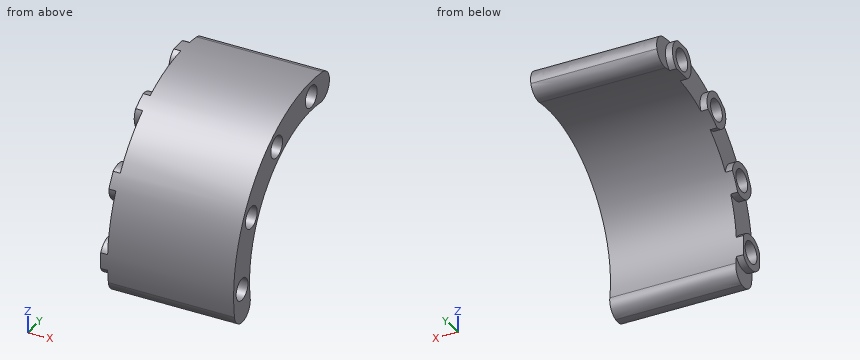
from build123d import *

# Parameters (mm, degrees)
SKETCH_1_R               = 41.5
SKETCH_1_R_2             = 33
EXTRUDE_1_DEPTH          = 38
SKETCH_2_R               = 3.15
CUT_EXTRUDE_1_DEPTH      = 70.91780889
PATTERN_CIRCULAR_1_COUNT = 4
PATTERN_CIRCULAR_1_ANGLE = 90
CUT_EXTRUDE_2_DEPTH      = 38
FILLET_START             = -1
FILLET_1_DEPTH           = 40
FILLET_2_DEPTH           = 38
SKETCH_4_OUTSIDE_W       = 69.583
SKETCH_4_OUTSIDE_H       = 69.583
SKETCH_4_OUTSIDE_R       = 5
CUT_EXTRUDE_3_DEPTH      = 2


with BuildPart() as part:
    # 草图1 → 凸台-拉伸1 (new body)
    with BuildSketch(Plane(origin=(0, 0, 0), x_dir=(0, 0, -1), z_dir=(1, 0, 0))):
        Circle(SKETCH_1_R)
        Circle(SKETCH_1_R_2, mode=Mode.SUBTRACT)
    extrude(amount=EXTRUDE_1_DEPTH)

    # 草图2 → 切除-拉伸1 (cut, through all)
    with BuildSketch(Plane.ZY):
        with Locations((37, 0)):
            Circle(SKETCH_2_R)
    cut_extrude_1 = extrude(amount=-CUT_EXTRUDE_1_DEPTH, mode=Mode.SUBTRACT)

    # 阵列(圆周)1: 切除-拉伸1 ×4 about axis
    pattern_circular_1_axis = Axis((0, 0, 0), (1, 0, 0))
    for i in range(1, PATTERN_CIRCULAR_1_COUNT):
        add(cut_extrude_1.rotate(pattern_circular_1_axis, i * PATTERN_CIRCULAR_1_ANGLE / (PATTERN_CIRCULAR_1_COUNT - 1)), mode=Mode.SUBTRACT)

    # 草图3 → 切除-拉伸2 (cut)
    with BuildSketch(Plane.ZY):
        with BuildLine():
            Line((40.085921791, 10.740990372), (0, 0))
            Line((0, 0), (-10.740990372, -40.085921791))
            ThreePointArc((-10.740990372, -40.085921791), (-29.344931419, 29.344931419), (40.085921791, 10.740990372))
        make_face()
    extrude(amount=-CUT_EXTRUDE_2_DEPTH, mode=Mode.SUBTRACT)

    # 圆角1: read off the stored shape, not the designer's step
    # 圆角1 outline → 圆角1 (cut)
    with BuildSketch(Plane.YZ.offset(FILLET_START)):
        with BuildLine():
            ThreePointArc((10.740990372, 40.085921791), (8.43291814, 40.634171477), (6.097289766, 41.049641381))
            add(Edge.make_bspline(
                [(6.097289766, 41.049641381), (7.224539758, 40.882205817), (8.479546293, 40.316443685), (9.579562271, 39.181662294), (10.053171447, 37.518946615), (9.578053286, 35.745781503)],
                knots=[0, 0, 0, 0, 0, 0, 0.528616925, 0.528616925, 0.528616925, 0.528616925, 0.528616925, 0.528616925], degree=5, weights=[1, 0.78855323, 0.632993631, 0.533321202, 0.489535944, 0.501637857]))
            Line((9.578053286, 35.745781503), (10.740990372, 40.085921791))
        make_face()
        with BuildLine():
            Line((8.541028488, 31.875552268), (9.578053286, 35.745781503))
            add(Edge.make_bspline(
                [(9.578053286, 35.745781503), (9.173304992, 34.235240304), (8.196828695, 33.153640695), (6.985664176, 32.610562324), (5.825288873, 32.496788788), (4.848447284, 32.641883508)],
                knots=[0.528616925, 0.528616925, 0.528616925, 0.528616925, 0.528616925, 0.528616925, 1, 1, 1, 1, 1, 1], degree=5, weights=[0.501637857, 0.512429484, 0.567661512, 0.667333941, 0.81144677, 1]))
            ThreePointArc((4.848447284, 32.641883508), (6.705693943, 32.31150985), (8.541028488, 31.875552268))
        make_face()
    extrude(amount=FILLET_1_DEPTH, mode=Mode.SUBTRACT)

    # 圆角2: read off the stored shape, not the designer's step
    # 圆角2 outline → 圆角2 (cut)
    with BuildSketch(Plane.YZ):
        with BuildLine():
            add(Edge.make_bspline(
                [(-41.049641381, -6.097289766), (-40.882205817, -7.224539758), (-40.316443685, -8.479546293), (-39.181662294, -9.579562271), (-37.518946615, -10.053171446), (-35.745781503, -9.578053286)],
                knots=[0, 0, 0, 0, 0, 0, 0.528616925, 0.528616925, 0.528616925, 0.528616925, 0.528616925, 0.528616925], degree=5, weights=[1, 0.78855323, 0.632993631, 0.533321202, 0.489535944, 0.501637857]))
            ThreePointArc((-41.049641381, -6.097289766), (-40.634171477, -8.43291814), (-40.085921791, -10.740990372))
            Line((-40.085921791, -10.740990372), (-35.745781503, -9.578053286))
        make_face()
        with BuildLine():
            add(Edge.make_bspline(
                [(-35.745781503, -9.578053286), (-34.235240304, -9.173304992), (-33.153640695, -8.196828695), (-32.610562324, -6.985664176), (-32.496788788, -5.825288873), (-32.641883508, -4.848447284)],
                knots=[0.528616925, 0.528616925, 0.528616925, 0.528616925, 0.528616925, 0.528616925, 1, 1, 1, 1, 1, 1], degree=5, weights=[0.501637857, 0.512429484, 0.567661512, 0.667333941, 0.81144677, 1]))
            Line((-35.745781503, -9.578053286), (-31.875552268, -8.541028488))
            ThreePointArc((-31.875552268, -8.541028488), (-32.31150985, -6.705693943), (-32.641883508, -4.848447284))
        make_face()
    extrude(amount=FILLET_2_DEPTH, mode=Mode.SUBTRACT)

    # 草图4 outside → 切除-拉伸3 (cut)
    with BuildSketch(Plane(origin=(0, 0, 0), x_dir=(0, 0, -1), z_dir=(1, 0, 0))):
        with Locations((-15.8885, -15.8885)):
            Rectangle(SKETCH_4_OUTSIDE_W, SKETCH_4_OUTSIDE_H)
        with Locations((-18.5, -32.04293994)):
            Circle(SKETCH_4_OUTSIDE_R, mode=Mode.SUBTRACT)
        with Locations((-37, 0)):
            Circle(SKETCH_4_OUTSIDE_R, mode=Mode.SUBTRACT)
        with Locations((0, -37)):
            Circle(SKETCH_4_OUTSIDE_R, mode=Mode.SUBTRACT)
        with Locations((-32.04293994, -18.5)):
            Circle(SKETCH_4_OUTSIDE_R, mode=Mode.SUBTRACT)
    extrude(amount=CUT_EXTRUDE_3_DEPTH, mode=Mode.SUBTRACT)


solid = part.part
Source: CAD feature listing. Evaluate the final solid. Frame: model axes, mm. Round coordinates to 2 decimals unless told otherwise and drop trailing zeros. Loops run counter-clockwise (first coordinate to the right, second up) from the corner with the lowest first, then second, coordinate; pieces in that order, holes last. Notation, with made-up numbers: (-6.5, 89.25) - (16.5, 89.25) arc R23 cw to (16.5, 110.25) - close; hole circle Ø7 at (-4.5, 20.5). An arc over 180 degrees is marked (long way). Write item = value, one per line. Start each with the question number.
(1) Section query C-C, the plane z = 16.5. Output: boundary loops of the cut face in (x, y), plus the area to 3 significant figures.
(2) Section query D-D, the plane x = 12. State how many separate pieces and enclosed holes the cut face has, plus the area to 3 significant figures.
(3) Ray query, line 1 along Y through (x, z) = (14, 21); line 2 along Y through (x, z) = (24, 18); line 3 along Z through (x, y) = (4, 1). Return the intervals inside material, ascending. Write a range as from..to.
(4) Pin query (flat end, axial travel): pin 1 (2 mm diameter, centred on y = -35.5, z = -7.5, fed in from -X); pin 2 (5.5 mm diameter, centred on y = 0, z = 37, fed in from -X); pin 3 (1.5 mm diameter, centred on x = 5, y = -28, fed in from +Z); pin 4 (12 mm diameter, centred on x = 15.5, y = -22, fed in from -Z). Return the tip coordinate at first contact, or that it passes through.
(5) Section query B-B, the plane z = 0. Output: boundary loops of the cut face in (x, y).
(6) Section query A-A, the plane y = 0. Output: boundary loops of the cut face in (x, z), plus the area to 3 significant figures.
Conclusion:
q1.outline = (0, -36.63) - (2, -36.63) - (2, -38.08) - (38, -38.08) - (38, -34.48) - (0, -34.48) - close; (0, -29.61) - (38, -29.61) - (38, -28.58) - (0, -28.58) - close
q1.area = 173 mm2
q2.separate_pieces = 1
q2.enclosed_holes = 4
q2.area = 523 mm2
q3.line_1 = -35.79..-33.96, -30.13..-25.46
q3.line_2 = -37.39..-35.15, -28.93..-27.66
q3.line_3 = 32.98..34.01, 39.99..41.49
q4.pin_1 = 2
q4.pin_2 = through
q4.pin_3 = 31.3
q4.pin_4 = 17.46
q5.outline = (0, -41.5) - (38, -41.5) - (38, -40.15) - (0, -40.15) - close; (0, -33.85) - (38, -33.85) - (38, -33) - (0, -33) - close
q6.outline = (0, 33) - (38, 33) - (38, 33.85) - (0, 33.85) - close; (0, 40.15) - (38, 40.15) - (38, 41.5) - (0, 41.5) - close
q6.area = 83.6 mm2
